```python
from build123d import *

# Parameters (mm, degrees)
SKETCH1_R           = 6.35
BOSS_EXTRUDE1_DEPTH = 6.35
SKETCH2_R           = 12.7
BOSS_EXTRUDE2_DEPTH = 3.175
BOSS_EXTRUDE3_DEPTH = 0.79375
CIRPATTERN1_COUNT   = 12
SKETCH4_R           = 3.175
CUT_EXTRUDE1_DEPTH  = 26.19931616


with BuildPart() as part:
    # Sketch1 → Boss-Extrude1 (new, symmetric)
    with BuildSketch(Plane(origin=(0, 0, 0), x_dir=(1, 0, 0), z_dir=(0, 1, 0))):
        with Locations(Location((0, 0, 0), (0, 0, 270))):
            Circle(SKETCH1_R)
    extrude(amount=BOSS_EXTRUDE1_DEPTH, both=True)

    # Sketch2 → Boss-Extrude2 (add, symmetric)
    with BuildSketch(Plane(origin=(0, 0, 0), x_dir=(1, 0, 0), z_dir=(0, 1, 0))):
        with Locations(Location((0, 0, 0), (0, 0, 270))):
            Circle(SKETCH2_R)
    extrude(amount=BOSS_EXTRUDE2_DEPTH, both=True)

    # Sketch3 → Boss-Extrude3 (add, symmetric)
    with BuildSketch(Plane(origin=(0, 0, 0), x_dir=(1, 0, 0), z_dir=(0, 1, 0))):
        with BuildLine():
            Line((-6.891666757, -13.415120246), (-3.89786608, -12.461780366))
            ThreePointArc((-3.89786608, -12.461780366), (-3.335621729, -12.448709767), (-2.855239137, -12.741151414))
            Line((-2.855239137, -12.741151414), (-0.739201637, -15.063668306))
            ThreePointArc((-0.739201637, -15.063668306), (-0.404051866, -15.304920203), (0, -15.390184127))
            Line((0, -15.390184127), (0, -12.7))
            Line((0, -12.7), (-6.35, -10.998522628))
            Line((-6.35, -10.998522628), (-7.695092063, -13.328290423))
            ThreePointArc((-7.695092063, -13.328290423), (-7.302540921, -13.456475632), (-6.891666757, -13.415120246))
        make_face()
    boss_extrude3 = extrude(amount=BOSS_EXTRUDE3_DEPTH, both=True)

    # CirPattern1: Boss-Extrude3 ×12 about axis
    cirpattern1_axis = Axis((0, 0, 0), (0, 1, 0))
    for i in range(1, CIRPATTERN1_COUNT):
        add(boss_extrude3.rotate(cirpattern1_axis, i * 360 / CIRPATTERN1_COUNT))

    # Sketch4 → Cut-Extrude1 (cut, through all)
    with BuildSketch(Plane(origin=(0, 6.35, 0), x_dir=(1, 0, 0), z_dir=(0, 1, 0))):
        with Locations(Location((0, 0, 0), (0, 0, 270))):
            Circle(SKETCH4_R)
    extrude(amount=-CUT_EXTRUDE1_DEPTH, mode=Mode.SUBTRACT)


solid = part.part
```
Design review of the part built by this model. Coordinates are the model's own, in mm. A direction names the side the tool comes from. Coordinates: 2 decimals unless noted, no trailing zeros. Order: outer loops, then holes, each group sorted by start corner. A loop starts at its lowest first (then second) coordinate and runs counter-clockwise, first axis right, second up. Notation, with made-up numbers: M 80.25,-5 L 93.25,-5 A36 cw 93.25,32 Z; hole C 7.25,54 d1. An arc over 180 degrees is marked long. Answer as a JSON object with one key per item and string values. Group by question number.
1) Add section A-A, the plane y = 2.5. Write out the cut boundary in (x, z) (3 decimals).
2) Add section C-C, the plane x = 14.5. Write out the cut boundary in (y, z), then the cut area to 3 significant figures.
3) For pin 1 (3 mm diameter, centred on x = -1, y = -5, fed in from -Z); pin 2 (8 mm diameter, centred on x = 5.5, z = 10.5, fed in from +Y) (3 decimals); pin 3 (5.5 mm diameter, centred on x = 0, z = 0, fed in from +Y); pin 4 (5 mm diameter, centred on x = -4, y = -4, fed in from +Z), all flat-tipped, find the tip position at first contact; note any pin that passes through.
4) Mouldability with a two-part tool opening along X and no side actions: class faces 5 (the cylindrical face through (-1.93, 0.09, -2.52)), 6 (the flat face through (6, -3.175, 3)), 7 (the flat face through (-5.416, 0.011, 12.945)), 8 (the flat face through (-12.93, 0.01, 5.37)) as pulls with the +X half, pulls with the -X half, needs draft (parallel to the pull), parting line crosses it, or undercut.
5) Tool access review of faces 1 (the flat face through (5.37, 0.01, 12.93)), 2 (the flat face through (-7, -0.794, -11)), 3 (the flat face through (12.945, 0.011, 5.416)), 4 (the cylindrical face through (-3.86, 4.78, -5.04)): name each direction out of +Z, -Z, +X, -X, +Y, -Y from which nothing blocks a thin tool from reaching the whole face with its end or side.
6) Wall thickness on L1, parallel to X at y = -1, z = 0 (3 decimals); L2, parallel to X at y = -3.75, z = 0 (3 decimals); L3, parallel to Y at x = 11, z = -6.5: over which ranges is each line inside the solid? List them lowest first.
7) Add section B-B, the plane x = -11.5. Write out the cut boundary in (y, z) (3 decimals), then the cut area to 3 significant figures.
Computed values:
{
 "1": {"outline": "C 0,0 d25.4; hole C 0,0 d6.35"},
 "2": {"outline": "M -0.79,-1.25 L 0.79,-1.25 L 0.79,1.25 L -0.79,1.25 Z", "area": "3.98 mm^2"},
 "3": {"pin 1": "stops at z = -6.35", "pin 2": "stops at y = 3.175", "pin 3": "passes through", "pin 4": "stops at z = 12.59"},
 "4": {"face 5": "undercut", "face 6": "needs draft", "face 7": "undercut", "face 8": "pulls with the -X half"},
 "5": {"face 1": "+Z, +Y, -Y", "face 2": "-Y", "face 3": "+X, +Y, -Y", "face 4": "+Y"},
 "6": {"L1": "x = -12.7 to -3.175, 3.175 to 12.7", "L2": "x = -6.35 to -3.175, 3.175 to 6.35", "L3": "y = -0.79 to 0.79"},
 "7": {"outline": "M -3.175,-5.389 L -0.794,-5.389 L -0.794,-8.429 L 0.794,-8.429 L 0.794,-5.389 L 3.175,-5.389 L 3.175,5.389 L 0.794,5.389 L 0.794,8.429 L -0.794,8.429 L -0.794,5.389 L -3.175,5.389 Z", "area": "78.1 mm^2"}
}
